from build123d import *

# Parameters (mm, degrees)
SKETCH1_W           = 40
SKETCH1_H           = 40
BOSS_EXTRUDE1_DEPTH = 40
CUT_EXTRUDE1_DEPTH  = 40
SKETCH3_W           = 2
SKETCH3_H           = 20
CUT_EXTRUDE2_DEPTH  = 40
CUT_EXTRUDE4_DEPTH  = 20
SKETCH9_W           = 18
SKETCH9_H           = 20
CUT_EXTRUDE7_DEPTH  = 1
SKETCH10_W          = 18
SKETCH10_H          = 20
CUT_EXTRUDE8_DEPTH  = 1


with BuildPart() as part:
    # Sketch1 → Boss-Extrude1 (new body)
    with BuildSketch(Plane.XY):
        with Locations((20, 20)):
            Rectangle(SKETCH1_W, SKETCH1_H)
    extrude(amount=BOSS_EXTRUDE1_DEPTH)

    # Sketch2 → Cut-Extrude1 (cut)
    with BuildSketch(Plane(origin=(0, 40, 0), x_dir=(1, 0, 0), z_dir=(0, 1, 0))):
        Polygon((10, -30), (0, -30), (0, -40), (30, -40), (30, -20), (10, -20), align=None)
        with BuildLine():
            Line((40, 0), (20, 0))
            ThreePointArc((20, 0), (34.142135624, -5.857864376), (40, -20))
            Line((40, -20), (40, 0))
        make_face()
        with BuildLine():
            Line((0, 0), (0, -20))
            ThreePointArc((0, -20), (5.857864376, -5.857864376), (20, 0))
            Line((20, 0), (0, 0))
        make_face()
    extrude(amount=-CUT_EXTRUDE1_DEPTH, mode=Mode.SUBTRACT)

    # Sketch3 → Cut-Extrude2 (cut)
    with BuildSketch(Plane(origin=(0, 0, 0), x_dir=(0, 0, -1), z_dir=(1, 0, 0))):
        with Locations((-1, 20)):
            Rectangle(SKETCH3_W, SKETCH3_H)
    extrude(amount=CUT_EXTRUDE2_DEPTH, mode=Mode.SUBTRACT)

    # Sketch5 → Cut-Extrude4 (cut)
    with BuildSketch(Plane(origin=(0, 30, 0), x_dir=(1, 0, 0), z_dir=(0, 1, 0))):
        with BuildLine():
            Line((28.717797887, -2), (28.717797887, -20))
            Line((28.717797887, -20), (11.282202113, -20))
            Line((11.282202113, -20), (11.282202113, -2))
            ThreePointArc((11.282202113, -2), (20, 0), (28.717797887, -2))
        make_face()
    extrude(amount=-CUT_EXTRUDE4_DEPTH, mode=Mode.SUBTRACT)

    # Sketch9 → Cut-Extrude7 (cut)
    with BuildSketch(Plane.ZY.offset(-28.717797887)):
        with Locations((11, 20)):
            Rectangle(SKETCH9_W, SKETCH9_H)
    extrude(amount=-CUT_EXTRUDE7_DEPTH, mode=Mode.SUBTRACT)

    # Sketch10 → Cut-Extrude8 (cut)
    with BuildSketch(Plane(origin=(11.282202113, 0, 0), x_dir=(0, 0, -1), z_dir=(1, 0, 0))):
        with Locations((-11, 20)):
            Rectangle(SKETCH10_W, SKETCH10_H)
    extrude(amount=-CUT_EXTRUDE8_DEPTH, mode=Mode.SUBTRACT)


solid = part.part
Input: part model. Units: mm. Frame: model coordinates. A direction names the side the tool comes from. Coordinates: 2 decimals unless noted, no trailing zeros. Loops run counter-clockwise (first coordinate to the right, second up) from the corner with the lowest first, then second, coordinate; pieces in that order, holes last.
(1) First-contact query: pin 1 Ø5 at (x, y) = (7.5, 29.5) entering from +Z; pin 2 Ø10 at (x, y) = (22.5, 26) entering from +Z; pin 3 Ø1.5 at (x, y) = (21, 34) entering from -Z. Flat tips, straight axial feed; report the tip coordinate or a pass-through.
(2) Section D-D on z = 16. Return the cut outline in (x, y), then the cut area to 3 significant figures.
(3) Section C-C on x = 15. Return the cut outline in (y, z), then the cut area to 3 significant figures.
(4) Material intervals for probe 1 along X at (y, z) = (4.5, 27); probe 2 along X at (y, z) = (38, 37); probe 3 along Z at (x, y) = (20, 31), sorted ascending.
(5) Section B-B on z = 27.5. Return the cut outline in (x, y).
(6) Pull-direction query (X, two-part tool) for faces 4 (the face through (0, 20, 25)), 5 (the face through (29.718, 20, 11)), 6 (the face through (40, 20, 30)), 7 (the face through (20, 0, 15)); classes: released by +X, released by -X, zero draft, split by the parting line, or undercut.
(7) Section A-A on y = 22. Return the cut outline in (x, z).
(8) Set-up query: faces 1 (the face through (5, 20, 30)), 2 (the face through (20, 30, 10)), 3 (the face through (20, 34, 20)). Return all of +Z, -Z, +X, -X, +Y, -Y with unobstructed straight access to the full face (end or side cutting, diameter ignored); none if empty.
Data:
1. pin 1: stops at z = 30
1. pin 2: stops at z = 20
1. pin 3: stops at z = 0
2. outline: (0.4, 0) - (39.6, 0) - (39.6, 40) - (0.4, 40) - close; hole (10.28, 10) - (29.72, 10) - (29.72, 30) - (10.28, 30) - close
2. area: 1,180 mm2
3. outline: (0, 0.64) - (10, 0.64) - (10, 20) - (0, 20) - close; (30, 0.64) - (40, 0.64) - (40, 20) - (30, 20) - close
3. area: 387 mm2
4. probe 1: x = 0 to 10, 30 to 40
4. probe 2: x = 30 to 40
4. probe 3: z = 0 to 20
5. outline: (0, 0) - (10, 0) - (10, 40) - (0, 40) - close; (30, 0) - (40, 0) - (40, 40) - (30, 40) - close
6. face 4: released by -X
6. face 5: undercut
6. face 6: released by +X
6. face 7: zero draft
7. outline: (0, 20) arc R20 ccw to (10.28, 2.52) - (10.28, 20) - (10, 20) - (10, 30) - (0, 30) - close; (29.72, 2.52) arc R20 ccw to (40, 20) - (40, 40) - (30, 40) - (30, 20) - (29.72, 20) - close
8. face 1: +Z, -X, +Y, -Y
8. face 2: +Z, -Z
8. face 3: +Z, +Y, -Y
